Solid Edge part; units mm, degrees
sketch "Sketch1" plane through (0, 0, -10) normal (0, 0, 1) x (1, 0, 0)
  line L0 (0, 4) -> (0, 38)
  line L1 (0, 38) -> (10, 38)
  line L2 (10, 38) -> (10, 0)
  line L3 (10, -38) -> (10, 0)
  line L4 (0, -38) -> (10, -38)
  line L5 (0, -4) -> (0, -38)
  arc A0 (0, -4) -> (0, 4) centre (0, 0) ccw
extrude "ExtrudedProtrusion_1" add sketch "Sketch1" along normal mid plane 16
sketch "Sketch2" plane through (0, 21, -10) normal (-1, 0, 0) x (0, 0, 1)
  circle A0 centre (0, 7.58) radius 4
  circle A1 centre (0, -49.58) radius 4
extrude "Cutout1" cut sketch "Sketch2" against normal through all
sketch "Sketch3" plane through (0, 21, -10) normal (-1, 0, 0) x (0, 0, 1)
  circle A0 centre (0, -14) radius 2.2
extrude "Cutout2" cut sketch "Sketch3" against normal through all
mirror "Mirror1" about plane through (0, 0, 0) normal (0, -1, 0) of "Cutout2"
Build history of the part. All positions in model axes, mm. Coordinates: 2 decimals unless noted, no trailing zeros. Order: outer loops, then holes, each group sorted by start corner. A loop starts at its lowest first (then second) coordinate and runs counter-clockwise, first axis right, second up.
Item 1: Mould opens along Z. For faces 1 (the cylindrical face through (4.93, -5.145, -8.817)), 2 (the flat face through (0, -21, -10)), 3 (the flat face through (5, 1, -18)) say: released by +Z, released by -Z, zero draft, split by the parting line, or undercut.
Filled in:
face 1: undercut
face 2: zero draft
face 3: released by -Z
Item 2: Drill centre lines: L1, parallel to Y at x = 7, z = -10; L2, parallel to Z at x = 4.5, y = -7; L3, parallel to Y at x = 2.75, z = -9.75. Where is each one in solid material? Low to high.
Filled in:
L1: y = -38 to -32.58, -24.58 to -9.2, -4.8 to 4.8, 9.2 to 24.58, 32.58 to 38
L2: z = -18 to -12.2, -7.8 to -2
L3: y = -38 to -32.57, -24.59 to -9.19, -4.81 to -2.9, 2.9 to 4.81, 9.19 to 24.59, 32.57 to 38
Item 3: Saw through at C-C on x = 8. List the corners of the cut face in (y, z), then the cut area to 3 significant figures.
Filled in:
outline: (-38, -18) - (38, -18) - (38, -2) - (-38, -2) - close; hole circle Ø8 at (-28.58, -10); hole circle Ø4.4 at (-7, -10); hole circle Ø4.4 at (7, -10); hole circle Ø8 at (28.58, -10)
area: 1,090 mm2
Item 4: Saw through at B-B on z = -10. List the corners of the cut face in (x, y).
Filled in:
outline: (0, -38) - (10, -38) - (10, -32.58) - (0, -32.58) - close; (0, -24.58) - (10, -24.58) - (10, -9.2) - (0, -9.2) - close; (0, -4.8) - (10, -4.8) - (10, 4.8) - (0, 4.8) - (0, 4) arc R4 cw to (0, -4) - close; (0, 9.2) - (10, 9.2) - (10, 24.58) - (0, 24.58) - close; (0, 32.58) - (10, 32.58) - (10, 38) - (0, 38) - close
Item 5: Saw through at D-D on y = 7. List the corners of the cut face in (x, z).
Filled in:
outline: (0, -18) - (10, -18) - (10, -12.2) - (0, -12.2) - close; (0, -7.8) - (10, -7.8) - (10, -2) - (0, -2) - close
Item 6: Saw through at A-A on x = 2.25. List the corners of the cut face in (y, z), then the cut area to 3 significant figures.
Filled in:
outline: (-38, -18) - (-3.31, -18) - (-3.31, -2) - (-38, -2) - close; (3.31, -18) - (38, -18) - (38, -2) - (3.31, -2) - close; hole circle Ø8 at (-28.58, -10); hole circle Ø4.4 at (-7, -10); hole circle Ø4.4 at (7, -10); hole circle Ø8 at (28.58, -10)
area: 979 mm2
